```python
from build123d import *

# Parameters (mm, degrees)
SKETCH1_W                    = 146
SKETCH1_H                    = 86
BOSS_EXTRUDE1_DEPTH          = 3
CSK_FOR_M3_SFHCS1_AT_2_COUNT = 2
CSK_FOR_M3_SFHCS1_AT_2_PITCH = 77
CSK_FOR_M3_SFHCS1_AT_3_COUNT = 2
CSK_FOR_M3_SFHCS1_AT_3_PITCH = 157.155973479
CSK_FOR_M3_SFHCS1_AT_4_COUNT = 2
CSK_FOR_M3_SFHCS1_AT_4_PITCH = 137
SKETCH5_R                    = 6.65
CUT_EXTRUDE1_DEPTH           = 14
SKETCH6_W                    = 6.85
SKETCH6_H                    = 19.5
SKETCH6_R                    = 1.5
BOSS_EXTRUDE2_DEPTH          = 10
SKETCH7_W                    = 7.05
SKETCH7_H                    = 2.001587211
SKETCH7_H_2                  = 2.00158721
CUT_EXTRUDE2_DEPTH           = 3
FILLET1_R                    = 5


with BuildPart() as part:
    # Sketch1 → Boss-Extrude1 (new body)
    with BuildSketch(Plane(origin=(0, 0, 0), x_dir=(1, 0, 0), z_dir=(0, 1, 0))):
        with Locations((6.693779904, -0.746411483)):
            Rectangle(SKETCH1_W, SKETCH1_H)
    extrude(amount=BOSS_EXTRUDE1_DEPTH)

    # Sketch3 → CSK for M3 SFHCS1 (revolve, cut)
    with BuildSketch(Plane(origin=(-61.806220096, 3, 39.246411483), x_dir=(0, 0, 1), z_dir=(1, 0, 0))):
        Polygon((0, 0), (0, 3), (1.7, 3), (1.7, 1.66), (3.36, 0), align=None)
    csk_for_m3_sfhcs1 = revolve(axis=Axis((-61.806220096, 9.35, 39.246411483), (0, -1, 0)), mode=Mode.SUBTRACT)

    # CSK for M3 SFHCS1 at 2: CSK for M3 SFHCS1 ×2
    with Locations(*[(0, 0, -i * CSK_FOR_M3_SFHCS1_AT_2_PITCH) for i in range(1, CSK_FOR_M3_SFHCS1_AT_2_COUNT)]):
        add(csk_for_m3_sfhcs1, mode=Mode.SUBTRACT)

    # CSK for M3 SFHCS1 at 3: CSK for M3 SFHCS1 ×2
    with Locations(*[Vector(0.8717454193280995, 0, -0.48995910429389533) * (i * CSK_FOR_M3_SFHCS1_AT_3_PITCH) for i in range(1, CSK_FOR_M3_SFHCS1_AT_3_COUNT)]):
        add(csk_for_m3_sfhcs1, mode=Mode.SUBTRACT)

    # CSK for M3 SFHCS1 at 4: CSK for M3 SFHCS1 ×2
    with Locations(*[(i * CSK_FOR_M3_SFHCS1_AT_4_PITCH, 0, 0) for i in range(1, CSK_FOR_M3_SFHCS1_AT_4_COUNT)]):
        add(csk_for_m3_sfhcs1, mode=Mode.SUBTRACT)

    # Sketch5 → Cut-Extrude1 (cut)
    with BuildSketch(Plane.XZ):
        with Locations(Location((6.693779904, 0.746411483, 0), (0, 0, 270))):
            Circle(SKETCH5_R)
    extrude(amount=-CUT_EXTRUDE1_DEPTH, mode=Mode.SUBTRACT)

    # Sketch6 → Boss-Extrude2 (add)
    # profile 1 of 2: a face of its own
    with BuildSketch(Plane.XZ):
        with Locations((-26.631220096, 0.746411483)):
            Rectangle(SKETCH6_W, SKETCH6_H)
        with Locations(Location((-27.471220096, 5.746411483, 0), (0, 0, 270))):
            Circle(SKETCH6_R, mode=Mode.SUBTRACT)
        with Locations(Location((-27.471220096, -4.253588517, 0), (0, 0, 270))):
            Circle(SKETCH6_R, mode=Mode.SUBTRACT)
    # profile 2 of 2: a face of its own
    with BuildSketch(Plane.XZ):
        with Locations((20.518779904, 0.746411483)):
            Rectangle(SKETCH6_W, SKETCH6_H)
        with Locations(Location((21.358779904, 5.746411483, 0), (0, 0, 270))):
            Circle(SKETCH6_R, mode=Mode.SUBTRACT)
        with Locations(Location((21.358779904, -4.253588517, 0), (0, 0, 270))):
            Circle(SKETCH6_R, mode=Mode.SUBTRACT)
    extrude(amount=BOSS_EXTRUDE2_DEPTH)

    # Sketch7 → Cut-Extrude2 (cut)
    with BuildSketch(Plane.XZ.offset(10)):
        with Locations((-26.731220096, 0.742822967)):
            Rectangle(SKETCH7_W, SKETCH7_H)
        with Locations((20.418779904, 0.746411483)):
            Rectangle(SKETCH7_W, SKETCH7_H_2)
    extrude(amount=-CUT_EXTRUDE2_DEPTH, mode=Mode.SUBTRACT)

    # Fillet1
    fillet1_edges = [part.edges().sort_by_distance(p)[0] for p in [
        (-66.306220096, 1.5, -42.253588517),
        (79.693779904, 1.5, -42.253588517),
        (79.693779904, 1.5, 43.746411483),
        (-66.306220096, 1.5, 43.746411483),
    ]]
    fillet(fillet1_edges, radius=FILLET1_R)


solid = part.part
```
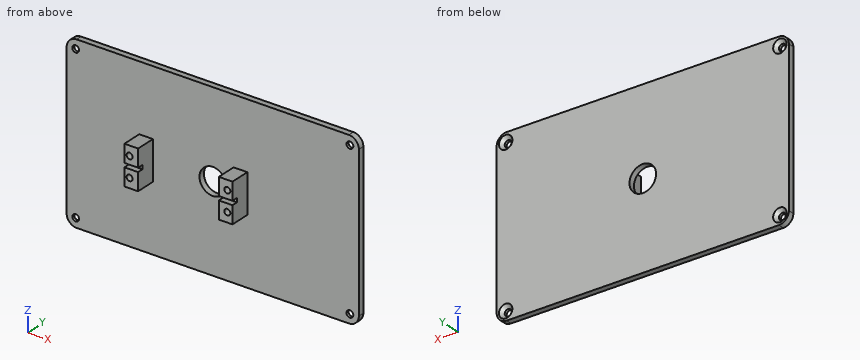
The listing builds one solid part. Answer for the finished solid, in the listing's coordinates (mm). Coordinates: 2 decimals unless noted, no trailing zeros. Write each loop counter-clockwise with the first axis right and the second up, starting at its lowest first coordinate (ties: lowest second). Pieces come first, ordered by that corner, then holes. Notation, with made-up numbers: (2.5, 68) - (9.5, 68) arc R25 ccw to (9.5, 89) - close; hole circle Ø7 at (1, 88). An arc over 180 degrees is marked (long way). One line per item, written item: value.
1) Find section A-A (y = -5.5). Give the vertices of the cut face in (x, z).
Geometry check:
outline: (-30.06, -9) - (-23.21, -9) - (-23.21, 10.5) - (-30.06, 10.5) - close; (17.09, -9) - (23.94, -9) - (23.94, 10.5) - (17.09, 10.5) - close; hole circle Ø3 at (-27.47, -4.25); hole circle Ø3 at (-27.47, 5.75); hole circle Ø3 at (21.36, -4.25); hole circle Ø3 at (21.36, 5.75)
2) Find section C-C (z = 18). Give the vertices of the cut face in (x, y), and give its area (3 significant figures).
Geometry check:
outline: (-66.31, 0) - (79.69, 0) - (79.69, 3) - (-66.31, 3) - close
area: 438 mm2
3) Each of these flat-tipped pins is pushed along its axis until it touches: pin 1 Ø1.6 at (x, z) = (19, 0.5) entering from -Y; pin 2 Ø2.5 at (x, y) = (-27.5, -9) entering from +Z; pin 3 Ø3.5 at (x, y) = (-25.5, -8.5) entering from -Z; pin 4 Ø8 at (x, z) = (28.5, 23) entering from -Y. Where does it stop, or does it pass through?
Geometry check:
pin 1: stops at y = -10
pin 2: stops at z = 10.5
pin 3: stops at z = -9
pin 4: stops at y = 0
4) Find section D-D (x = 61.5). Give the vertices of the cut face in (y, z).
Geometry check:
outline: (0, -42.25) - (3, -42.25) - (3, 43.75) - (0, 43.75) - close
5) Consider line 1 along X through (y, z) = (-4.5, -1.5); line 2 along Y through (x, z) = (34.5, 6); line 3 along X through (y, z) = (0.5, 3). Determine where each line is inside the solid, lowest interval first. Write a range as from..to.
Geometry check:
line 1: x = -30.06..-23.21, 17.09..23.94
line 2: y = 0..3
line 3: x = -66.31..0.44, 12.95..79.69
6) Find section B-B (x = 5). Give the vertices of the cut face in (y, z).
Geometry check:
outline: (0, -42.25) - (3, -42.25) - (3, -5.68) - (0, -5.68) - close; (0, 7.18) - (3, 7.18) - (3, 43.75) - (0, 43.75) - close
